Can you work these out from the model? Positions are in its coordinate system, mm. Face numbers are marked on the shaded views. A direction names the side the tool comes from. Round coordinates to 2 decimals unless told otherwise and drop trailing zeros. Loops run counter-clockwise (first coordinate to the right, second up) from the corner with the lowest first, then second, coordinate; pieces in that order, holes last. Notation, with made-up numbers: M 52,54 L 76,54 A17 ccw 76,77 Z; hole C 72,43 d7. An arc over 180 degrees is marked long. Use a Markdown table: item, result. Add a question column.
```python
from build123d import *

# Parameters (mm, degrees)
F0_R     = 1.905
F1_DEPTH = 1.27
F3_DEPTH = 10.16
F4_W     = 3.81
F4_H     = 11.43
F5_DEPTH = 15.24
F6_R     = 3.175
F7_DEPTH = 25.4
F8_SIZE  = 2.54


with BuildPart() as f1:
    # F0 (on Top) → F1 (new body)
    with BuildSketch(Plane.XY):
        with BuildLine():
            Line((16.51, 6.561151), (-16.51, 6.561151))
            ThreePointArc((-16.51, 6.561151), (-20.102102, 5.073253), (-21.59, 1.481151))
            Line((-21.59, 1.481151), (-21.59, -8.500309))
            Line((-21.59, -8.500309), (-20.149636, -8.500309))
            ThreePointArc((-20.149636, -8.500309), (0, 2.751151), (20.149636, -8.500309))
            Line((20.149636, -8.500309), (21.59, -8.500309))
            Line((21.59, -8.500309), (21.59, 1.481151))
            ThreePointArc((21.59, 1.481151), (20.102102, 5.073253), (16.51, 6.561151))
        make_face()
        with Locations((-16.51, 1.481151)):
            Circle(F0_R, mode=Mode.SUBTRACT)
        with Locations((16.51, 1.481151)):
            Circle(F0_R, mode=Mode.SUBTRACT)
        with BuildLine():
            Line((-20.149636, -8.500309), (-21.59, -8.500309))
            Line((-21.59, -8.500309), (-21.59, -11.218849))
            ThreePointArc((-21.59, -11.218849), (-20.914037, -9.836151), (-20.149636, -8.500309))
        make_face()
        with BuildLine():
            Line((21.59, -11.218849), (21.59, -8.500309))
            Line((21.59, -8.500309), (20.149636, -8.500309))
            ThreePointArc((20.149636, -8.500309), (20.914037, -9.836151), (21.59, -11.218849))
        make_face()
    extrude(amount=F1_DEPTH)

    # F2 (on face) → F3 (join)
    with BuildSketch(Plane.XY.offset(1.27)):
        with BuildLine():
            Line((21.59, -8.781116), (21.59, 1.481151))
            ThreePointArc((21.59, 1.481151), (20.102102, 5.073253), (16.51, 6.561151))
            Line((16.51, 6.561151), (-16.51, 6.561151))
            ThreePointArc((-16.51, 6.561151), (-20.102102, 5.073253), (-21.59, 1.481151))
            Line((-21.59, 1.481151), (-21.59, -8.781116))
            Line((-21.59, -8.781116), (-20.32, -8.781116))
            Line((-20.32, -8.781116), (-20.32, 1.481151))
            ThreePointArc((-20.32, 1.481151), (-19.204077, 4.175228), (-16.51, 5.291151))
            Line((-16.51, 5.291151), (16.51, 5.291151))
            ThreePointArc((16.51, 5.291151), (19.204077, 4.175228), (20.32, 1.481151))
            Line((20.32, 1.481151), (20.32, -8.781116))
            Line((20.32, -8.781116), (21.59, -8.781116))
        make_face()
    extrude(amount=F3_DEPTH)

    # F4 (on face) → F5 (join)
    with BuildSketch(Plane(origin=(0, 6.561151, 0), x_dir=(-1, 0, 0), z_dir=(0, 1, 0))):
        with Locations((6.985, 5.715)):
            Rectangle(F4_W, F4_H)
    extrude(amount=F5_DEPTH)

    # F6 (on face) → F7 (cut)
    with BuildSketch(Plane.YZ.offset(-5.08)):
        with BuildLine():
            ThreePointArc((21.801151, 5.715), (20.127266, 1.673885), (16.086151, 0))
            Line((16.086151, 0), (21.801151, 0))
            Line((21.801151, 0), (21.801151, 5.715))
        make_face()
        with Locations((16.086151, 5.715)):
            Circle(F6_R)
        with BuildLine():
            ThreePointArc((16.086151, 11.43), (20.127266, 9.756115), (21.801151, 5.715))
            Line((21.801151, 5.715), (21.801151, 11.43))
            Line((21.801151, 11.43), (16.086151, 11.43))
        make_face()
    extrude(amount=-F7_DEPTH, mode=Mode.SUBTRACT)

    # F8
    f8_edges = [f1.edges().sort_by_distance(p)[0] for p in [
        (-5.08, 6.561151, 5.715),
        (-8.89, 6.561151, 5.715),
    ]]
    chamfer(f8_edges, length=F8_SIZE)


solid = f1.part
```
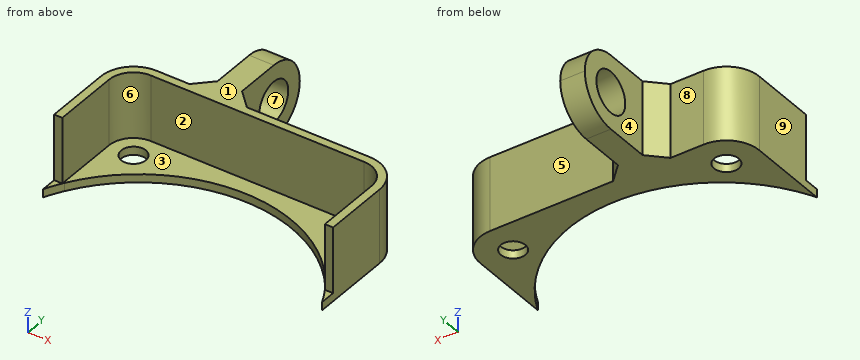
(1) If I drill on probe 1 along X at (y, z) = (-6, 9); probe 2 along Y at (x, z) = (3, 2.25); probe 3 along X at (y, z) = (13, 3), over which ranges is the centre line in solid material (lowest first)? Write a range as [from, to].
(2) Suppose I cut it at B-B on z = 7.75. List the corners of the cut face in (x, y) for me.
(3) I'm going to push flat-ended pins straight in: pin 1 (1 mm diameter, centred on x = 13.5, z = 6, fed in from +Y); pin 2 (0.6 mm diameter, centred on x = 21, z = 5.5, fed in from -Y); pin 3 (3 mm diameter, centred on y = 10, z = 3.5, fed in from -X); pin 4 (1.5 mm diameter, centred on x = 15.5, y = 7, fed in from -Z). Where does each tip first touch, or does it pass through?
(4) On a 3-axis mill with a long thin cutter (end or side, diameter ignored), from which of +Z, -Z, +X, -X, +Y, -Y can I reach the whole of each face in a straight line? I mean the marked faces 5, 6, 7, 8 and 9. Say none if no direction works.
(5) Suppose I cut it at D-D on x = 11. List the corners of the cut face in (y, z) for me, and give its area (3 significant figures).
(6) Suppose I cut it at A-A on y = -5. List the corners of the cut face in (x, z) for me.
(7) Thinking about a two-plate mould opening in X: for the marked faces 1, 2, 3 and 4, which applies, released by +X, released by -X, zero draft, split by the parting line, or undercut?
(8) Suppose I cut it at C-C on x = -7. List the corners of the cut face in (y, z) for me (3 decimals).
Results below:
| question | item | result |
|---|---|---|
| 1 | probe 1 | x = [-21.59, -20.32], [20.32, 21.59] |
| 1 | probe 2 | y = [5.29, 6.56] |
| 1 | probe 3 | x = [-8.89, -5.08] |
| 2 | outline | M -21.59,-8.78 L -20.32,-8.78 L -20.32,1.48 A3.81 cw -16.51,5.29 L 16.51,5.29 A3.81 cw 20.32,1.48 L 20.32,-8.78 L 21.59,-8.78 L 21.59,1.48 A5.08 ccw 16.51,6.56 L -2.54,6.56 L -5.08,9.1 L -5.08,13.65 L -8.89,13.65 L -8.89,9.1 L -11.43,6.56 L -16.51,6.56 A5.08 ccw -21.59,1.48 Z; M -8.89,18.52 L -5.08,18.52 L -5.08,21.43 L -8.89,21.43 Z |
| 3 | pin 1 | stops at y = 6.56 |
| 3 | pin 2 | stops at y = -8.78 |
| 3 | pin 3 | stops at x = -9.49 |
| 3 | pin 4 | stops at z = 0 |
| 4 | face 5 | +Z, -Z, +X, +Y |
| 4 | face 6 | +Z, -Y |
| 4 | face 7 | +X, -X |
| 4 | face 8 | +Z, -Z, -X, +Y |
| 4 | face 9 | +Z, -Z, -X, +Y, -Y |
| 5 | outline | M 0.04,0 L 6.56,0 L 6.56,11.43 L 5.29,11.43 L 5.29,1.27 L 0.04,1.27 Z |
| 5 | area | 21.2 mm² |
| 6 | outline | M -21.59,0 L -17.52,0 L -17.52,1.27 L -20.32,1.27 L -20.32,11.43 L -21.59,11.43 Z; M 17.52,0 L 21.59,0 L 21.59,11.43 L 20.32,11.43 L 20.32,1.27 L 17.52,1.27 Z |
| 7 | face 1 | zero draft |
| 7 | face 2 | undercut |
| 7 | face 3 | undercut |
| 7 | face 4 | released by -X |
| 8 | outline | M 1.692,0 L 16.086,0 A5.715 ccw 21.801,5.715 A5.715 ccw 16.086,11.43 L 5.291,11.43 L 5.291,1.27 L 1.692,1.27 Z; hole C 16.086,5.715 d6.35 |
